Source: CAD feature listing. Evaluate the final solid. Frame: model axes, mm. A direction names the side the tool comes from. Coordinates: 2 decimals unless noted, no trailing zeros. Write each loop counter-clockwise with the first axis right and the second up, starting at its lowest first coordinate (ties: lowest second). Pieces come first, ordered by that corner, then holes. Notation, with made-up numbers: (14.5, 10) - (49.5, 10) arc R30 ccw to (49.5, 42) - close; hole circle Ø9 at (-33.75, -13). An arc over 180 degrees is marked (long way). One line per question, with ' | ' between items.
Autodesk Inventor part; units mm, degrees
ref_plane "YZ Plane" through (0, 0, 0) normal (1, 0, 0) x (0, 1, 0)
ref_plane "XZ Plane" through (0, 0, 0) normal (0, 1, 0) x (-1, 0, 0)
ref_plane "XY Plane" through (0, 0, 0) normal (0, 0, 1) x (1, 0, 0)
sketch "Sketch1" plane through (0, 0, 0) normal (0, 0, 1) x (1, 0, 0)
  circle A0 centre (0, 0) radius 127
  dimension "d0" = 254
extrude "Extrusion1" add sketch "Sketch1" along normal blind 25.4
sketch "Sketch2" plane through (0, 0, 25.4) normal (0, 0, 1) x (1, 0, 0)
  circle A0 centre (0, 0) radius 56.134
  dimension "d4" = 112.268
extrude "Extrusion2" cut sketch "Sketch2" against normal blind 25.4
sketch "Sketch3" plane through (0, 0, 25.4) normal (0, 0, 1) x (1, 0, 0)
  circle A0 centre (76.2, 50.8) radius 12.7
  point P0 (0, 0)
  dimension "d7" = 25.4
  dimension "d8" = 50.8
  dimension "d9" = 76.2
extrude "Extrusion3" add sketch "Sketch3" along normal blind 25.4
properties part number "Manivela"
Item 1: Cut plane B-B on y = -5.5. Return loops of the section in (x, z).
Check sheet entries:
outline: (-126.88, 0) - (-55.86, 0) - (-55.86, 25.4) - (-126.88, 25.4) - close; (55.86, 0) - (126.88, 0) - (126.88, 25.4) - (55.86, 25.4) - close
Item 2: Pin query (flat end, axial travel): pin 1 Ø1.5 at (y, z) = (-40.5, 25) entering from -X; pin 2 Ø12 at (y, z) = (-98, 28) entering from -X; pin 3 Ø4 at (x, y) = (95.5, 7.5) entering from -Z; pin 4 Ø4 at (x, y) = (-53, -68.5) entering from +Z. Return the tip coordinate at first contact, or that it passes through.
Check sheet entries:
pin 1: x = -120.62 | pin 2: x = -86.92 | pin 3: z = 0 | pin 4: z = 25.4
Item 3: Cut plane D-D on z = 5. Return loops of the section in (x, y).
Check sheet entries:
outline: circle Ø254 at (0, 0); hole circle Ø112.27 at (0, 0)
Item 4: Cut plane A-A on x = 0. Return loops of the section in (y, z).
Check sheet entries:
outline: (-127, 0) - (-56.13, 0) - (-56.13, 25.4) - (-127, 25.4) - close; (56.13, 0) - (127, 0) - (127, 25.4) - (56.13, 25.4) - close
Item 5: Access query for faces 1 (the face through (66.1, 58.5, 37.9)), 2 (the face through (-27.53, 123.98, 12.52)). Directions: +Z, -Z, +X, -X, +Y, -Y. A direction counts if a zero-diameter tool reaches every point of the face in a straight line with its end or side. Return the directions, or none.
Check sheet entries:
face 1: +Z | face 2: +Z, -Z
Item 6: Cut plane C-C on x = 76.2. Return loops of the section in (y, z).
Check sheet entries:
outline: (-101.6, 0) - (101.6, 0) - (101.6, 25.4) - (63.5, 25.4) - (63.5, 50.8) - (38.1, 50.8) - (38.1, 25.4) - (-101.6, 25.4) - close
Item 7: Ray query, line 1 along Y through (x, z) = (0, 11); line 2 along Z through (x, y) = (33, -108.5); line 3 along Y through (x, z) = (3, 23). Return the intervals inside material, ascending. Write a range as [from, to].
Check sheet entries:
line 1: [-127, -56.13], [56.13, 127] | line 2: [0, 25.4] | line 3: [-126.96, -56.05], [56.05, 126.96]
